Geometry check sheet. Reference: the model listing, model coordinates, mm. Face numbers are marked on the shaded views. A direction names the side the tool comes from. Give positions to 0.01 mm unless a question says otherwise; leave off trailing zeros. Write each loop counter-clockwise with the first axis right and the second up, starting at its lowest first coordinate (ties: lowest second). Pieces come first, ordered by that corner, then holes. Notation, with made-up numbers: (-23.75, 37.25) -> (-15.75, 37.25) arc R28 ccw to (-15.75, 60.25) -> close; hole circle Ø11 at (59.5, 87). An arc over 180 degrees is marked (long way). One line per item, written item: value.
from build123d import *

# Parameters (mm, degrees)
SKETCH1_W           = 15
SKETCH1_H           = 26
BOSS_EXTRUDE1_DEPTH = 6
SKETCH2_R           = 1
BOSS_EXTRUDE2_DEPTH = 5
SKETCH3_R           = 1
BOSS_EXTRUDE3_DEPTH = 5
SKETCH5_R           = 3.375
BOSS_EXTRUDE4_DEPTH = 12.125


with BuildPart() as part:
    # Sketch1 → Boss-Extrude1 (new body)
    with BuildSketch(Plane.XY):
        Rectangle(SKETCH1_W, SKETCH1_H)
    extrude(amount=BOSS_EXTRUDE1_DEPTH)

    # Sketch2 → Boss-Extrude2 (add)
    with BuildSketch(Plane(origin=(0, 13, 0), x_dir=(1, 0, 0), z_dir=(0, 1, 0))):
        with Locations(Location((-6.25, -3, 0), (0, 0, 90))):
            Circle(SKETCH2_R)
        with Locations(Location((6.25, -3, 0), (0, 0, 90))):
            Circle(SKETCH2_R)
    extrude(amount=BOSS_EXTRUDE2_DEPTH)

    # Sketch3 → Boss-Extrude3 (add)
    with BuildSketch(Plane.XZ.offset(13)):
        with Locations(Location((0, 3, 0), (0, 0, 90))):
            Circle(SKETCH3_R)
        with Locations(Location((5, 3, 0), (0, 0, 90))):
            Circle(SKETCH3_R)
        with Locations(Location((-5, 3, 0), (0, 0, 90))):
            Circle(SKETCH3_R)
    extrude(amount=BOSS_EXTRUDE3_DEPTH)

    # Sketch5 → Boss-Extrude4 (add)
    with BuildSketch(Plane(origin=(0, 13, 0), x_dir=(1, 0, 0), z_dir=(0, 1, 0))):
        with Locations(Location((0, -3, 0), (0, 0, 62.733955549))):
            Circle(SKETCH5_R)
    extrude(amount=BOSS_EXTRUDE4_DEPTH)


solid = part.part
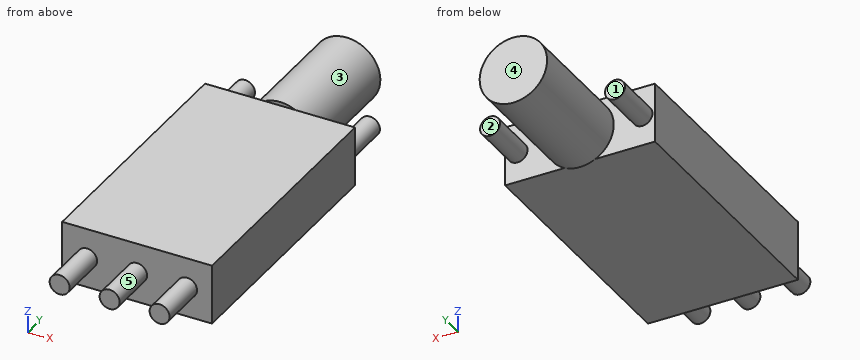
1) Depth check by flat-ended pin: pin 1 Ø1.6 at (x, z) = (-6.5, 3) entering from +Y; pin 2 Ø1.5 at (y, z) = (13.5, 5) entering from +X. Enter the tip coordinate at first touch or a pass-through.
Verdict:
pin 1: y = 18
pin 2: x = 7.5
2) Tool access check on the marked faces 1, 2, 3, 4 and 5. Record the directions out of +Z, -Z, +X, -X, +Y, -Y that give a thin tool (end or side, any length) a straight path to the whole face; none if there is none.
Verdict:
face 1: +Z, -Z, -X, +Y
face 2: +Z, -Z, +X, +Y
face 3: +Y
face 4: +Z, -Z, +X, -X, +Y
face 5: -Y
3) Sectioned sample at B-B on x = 0. Record the cut outline in (y, z) (3 decimals), plus the area to 3 significant figures.
Verdict:
outline: (-18, 2) -> (-13, 2) -> (-13, 0) -> (13, 0) -> (13, -0.375) -> (25.125, -0.375) -> (25.125, 6.375) -> (13, 6.375) -> (13, 6) -> (-13, 6) -> (-13, 4) -> (-18, 4) -> close
area: 248 mm^2
4) Sectioned sample at C-C on y = 14. Record the cut outline in (x, z) (3 decimals), plus the area to 3 significant figures.
Verdict:
outline: circle Ø2 at (-6.25, 3); circle Ø6.75 at (0, 3); circle Ø2 at (6.25, 3)
area: 42.1 mm^2
5) Sectioned sample at A-A on z = 3. Record the cut outline in (x, y) (3 decimals).
Verdict:
outline: (-7.5, -13) -> (-6, -13) -> (-6, -18) -> (-4, -18) -> (-4, -13) -> (-1, -13) -> (-1, -18) -> (1, -18) -> (1, -13) -> (4, -13) -> (4, -18) -> (6, -18) -> (6, -13) -> (7.5, -13) -> (7.5, 13) -> (7.25, 13) -> (7.25, 18) -> (5.25, 18) -> (5.25, 13) -> (3.375, 13) -> (3.375, 25.125) -> (-3.375, 25.125) -> (-3.375, 13) -> (-5.25, 13) -> (-5.25, 18) -> (-7.25, 18) -> (-7.25, 13) -> (-7.5, 13) -> close
6) Scan lines: probe 1 along Z at (x, y) = (2, 1); probe 2 along Y at (x, z) = (3.25, 3.75) (3 decimals); probe 3 along Y at (x, z) = (-4.25, 5.75). Record each from-to range of solid material in increasing order.
Verdict:
probe 1: 0 to 6
probe 2: -13 to 25.125
probe 3: -13 to 13
7) Sectioned sample at D-D on y = 21. Record the cut outline in (x, z) (3 decimals), plus the area to 3 significant figures.
Verdict:
outline: circle Ø6.75 at (0, 3)
area: 35.8 mm^2
